Geometry: final body of the model. Coordinates: model frame, mm. Give positions to 0.01 mm unless a question says otherwise; leave off trailing zeros. Loops run counter-clockwise (first coordinate to the right, second up) from the corner with the lowest first, then second, coordinate; pieces in that order, holes last.
from build123d import *

# Parameters (mm, degrees)
SKETCH_1_R          = 35
EXTRUDE_1_DEPTH     = 6
SKETCH_2_R          = 21
SKETCH_2_R_2        = 2.5
SKETCH_2_R_3        = 2.1
CUT_EXTRUDE_1_DEPTH = 10
CHAMFER_1_SIZE      = 2


with BuildPart() as part:
    # Эскиз1 → Бобышка-Вытянуть1 (new body)
    with BuildSketch(Plane(origin=(0, 0, 0), x_dir=(1, 0, 0), z_dir=(0, 1, 0))):
        with Locations(Location((0, 0, 0), (0, 0, 270))):
            Circle(SKETCH_1_R)
    extrude(amount=EXTRUDE_1_DEPTH)

    # Эскиз2 → Вырез-Вытянуть1 (cut)
    with BuildSketch(Plane(origin=(0, 6, 0), x_dir=(1, 0, 0), z_dir=(0, 1, 0))):
        with Locations(Location((0, 0, 0), (0, 0, 270))):
            Circle(SKETCH_2_R)
        with Locations(Location((0, 26, 0), (0, 0, 270))):
            Circle(SKETCH_2_R_2)
        with Locations(Location((0, -26, 0), (0, 0, 270))):
            Circle(SKETCH_2_R_2)
        with Locations(Location((26, 0, 0), (0, 0, 270))):
            Circle(SKETCH_2_R_2)
        with Locations(Location((-26, 0, 0), (0, 0, 270))):
            Circle(SKETCH_2_R_2)
        with Locations(Location((-22.273863607, 22.273863607, 0), (0, 0, 270))):
            Circle(SKETCH_2_R_3)
        with Locations(Location((-22.273863607, -22.273863607, 0), (0, 0, 270))):
            Circle(SKETCH_2_R_3)
        with Locations(Location((22.273863607, -22.273863607, 0), (0, 0, 270))):
            Circle(SKETCH_2_R_3)
        with Locations(Location((22.273863607, 22.273863607, 0), (0, 0, 270))):
            Circle(SKETCH_2_R_3)
    extrude(amount=-CUT_EXTRUDE_1_DEPTH, mode=Mode.SUBTRACT)

    # Фаска1
    chamfer_1_edges = [part.edges().sort_by_distance(p)[0] for p in [
        (0, 0, -28.5),
        (0, 0, 23.5),
        (26, 0, -2.5),
        (-26, 0, -2.5),
    ]]
    chamfer(chamfer_1_edges, length=CHAMFER_1_SIZE)


solid = part.part
Item 1: Draft query along Z for faces 1 (the face through (-15, 0, 15)), 2 (the face through (24.045, 3.042, 23.403)), 3 (the face through (-21, 3, -28)). Return one class per face: +Z half, -Z half, draft (parallel to the pull), parting line (faces both ways), or undercut.
Values follow:
face 1: draft
face 2: undercut
face 3: parting line
Item 2: Ray query, probe 1 along X at (y, z) = (4.7, 0); probe 2 along Z at (x, y) = (1, 2.55); probe 3 along X at (y, z) = (2.4, -1.5). Return the intervals inside material, ascending.
Values follow:
probe 1: x = -35 to -28.5, -23.5 to -21, 21 to 23.5, 28.5 to 35
probe 2: z = -34.99 to -28.29, -23.71 to -20.98, 20.98 to 23.71, 28.29 to 34.99
probe 3: x = -34.97 to -28, -24 to -20.95, 20.95 to 24, 28 to 34.97
Item 3: Section query A-A on x = 0. Return loops of the section in (y, z).
Values follow:
outline: (0, -35) - (6, -35) - (6, -28.5) - (2, -28.5) - (0, -30.5) - close; (0, -21.5) - (2, -23.5) - (6, -23.5) - (6, -21) - (0, -21) - close; (0, 21) - (6, 21) - (6, 23.5) - (2, 23.5) - (0, 21.5) - close; (0, 30.5) - (2, 28.5) - (6, 28.5) - (6, 35) - (0, 35) - close
Item 4: Section query B-B on z = -26. Return loops of the section in (x, y).
Values follow:
outline: (-23.43, 0) - (-4.5, 0) - (-2.5, 2) - (-2.5, 6) - (-23.43, 6) - close; (2.5, 2) - (4.5, 0) - (23.43, 0) - (23.43, 6) - (2.5, 6) - close
Item 5: Section query C-C on y = 2.85. Give the number of separate pieces and of enclosed holes in the cut face, plus the area to 3 significant figures.
Values follow:
separate pieces: 1
enclosed holes: 9
area: 2,330 mm2
Item 6: Pin query (flat end, axial travel): pin 1 (3.5 mm diameter, centred on x = 22.27, z = -22.27, fed in from -Y); pin 2 (6.5 mm diameter, centred on x = 0, z = -26, fed in from +Y); pin 3 (3 mm diameter, centred on x = 21.5, y = 4, fed in from -Z); pin 4 (1.5 mm diameter, centred on y = 5, z = -14.5, fed in from -X). Return the tip coordinate at first contact, or that it passes through.
Values follow:
pin 1: passes through
pin 2: stops at y = 6
pin 3: stops at z = -28.72
pin 4: stops at x = -32.19
Item 7: Section query D-D on x = 26. Return loops of the section in (y, z), plus the area to 3 significant figures.
Values follow:
outline: (0, -23.43) - (6, -23.43) - (6, -2.5) - (2, -2.5) - (0, -4.5) - close; (0, 4.5) - (2, 2.5) - (6, 2.5) - (6, 23.43) - (0, 23.43) - close
area: 247 mm2
